Source: CAD feature listing. Evaluate the final solid. Frame: model axes, mm. Face numbers are marked on the shaded views. A direction names the side the tool comes from. Coordinates: 2 decimals unless noted, no trailing zeros. Write each loop counter-clockwise with the first axis right and the second up, starting at its lowest first coordinate (ties: lowest second). Pieces come first, ordered by that corner, then holes. Notation, with made-up numbers: (24.25, 86) -> (37.25, 86) arc R23 ccw to (37.25, 100) -> close; hole circle Ø3 at (12.5, 4). An arc over 180 degrees is marked (long way). One line per item, written item: value. Start each with the question number.
1. Mould query, pull axis Y, two halves, no side actions, for the marked faces 1, 2 and 3. Classes: released by +Y, released by -Y, zero draft, split by the parting line, or undercut.
2. Section query D-D, the plane z = 2.5. Output: boundary loops of the cut face in (x, y), and give its area (3 significant figures).
3. Section query C-C, the plane y = -0.9. Output: boundary loops of the cut face in (x, z), and give its area (3 significant figures).
4. Section query A-A, the plane z = 6.75. Output: boundary loops of the cut face in (x, y).
5. Line query: line 1 (Y direction, x = 0, z = 1.95); line 2 (Z direction, x = 1.1, y = -0.1); line 3 (X direction, y = 0.05, z = 3.75). Output: solid intervals per line, ascending.
6. Section query B-B, the plane x = -0.75. Output: boundary loops of the cut face in (y, z).
7. Access query for the marked faces 4, 5 and 6. Directions: +Z, -Z, +X, -X, +Y, -Y. A direction counts if a zero-diameter tool reaches every point of the face in a straight line with its end or side. Return the directions, or none.
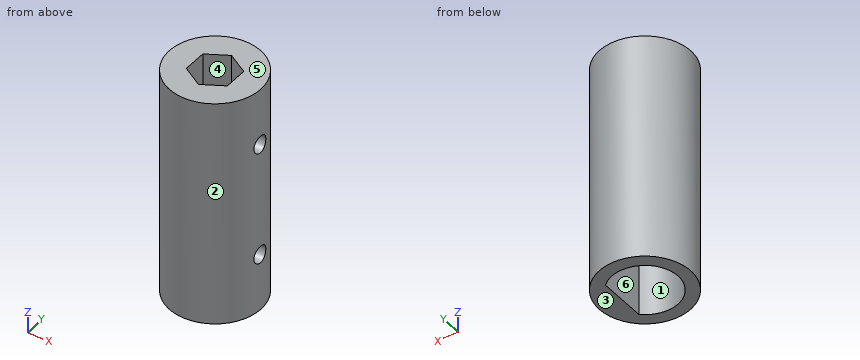
from build123d import *

# Parameters (mm, degrees)
MOTORSKE_R      = 2
MOTOR_DEPTH     = 5
AXISSKE_R       = 2
AXIS_DEPTH      = 5
SCREWHOLESKE_R  = 0.376260287
SCREWHOLE_DEPTH = 11.392304845


with BuildPart() as part:
    # MotorSke → Motor (new body)
    with BuildSketch(Plane.XY):
        Circle(MOTORSKE_R)
        with BuildLine():
            Line((1, 1.05), (1, -1.05))
            ThreePointArc((1, -1.05), (-1.45, 0), (1, 1.05))
        make_face(mode=Mode.SUBTRACT)
    extrude(amount=MOTOR_DEPTH)

    # AxisSke → Axis (add)
    with BuildSketch(Plane.XY.offset(5)):
        Circle(AXISSKE_R)
        Polygon((0, -1.039230485), (0.9, -0.519615242), (0.9, 0.519615242), (0, 1.039230485), (-0.9, 0.519615242), (-0.9, -0.519615242), align=None, mode=Mode.SUBTRACT)
    extrude(amount=AXIS_DEPTH)

    # ScrewHoleSke → ScrewHole (cut, through all)
    with BuildSketch(Plane(origin=(0, 0, 0), x_dir=(0, 0, -1), z_dir=(1, 0, 0))):
        with Locations(Location((-7.5, 0, 0), (0, 0, 180))):
            Circle(SCREWHOLESKE_R)
        with Locations(Location((-2.5, 0, 0), (0, 0, 180))):
            Circle(SCREWHOLESKE_R)
    extrude(amount=SCREWHOLE_DEPTH, mode=Mode.SUBTRACT)


solid = part.part
Computed values:
1. face 1: undercut
1. face 2: split by the parting line
1. face 3: zero draft
2. outline: (1, -1.05) arc R1.45 cw (long way) to (1, 1.05) -> (1, 0.38) -> (1.96, 0.38) arc R2 ccw (long way) to (1.96, -0.38) -> (1, -0.38) -> close
2. area: 5.87 mm²
3. outline: (-1.79, 0) -> (-1.14, 0) -> (-1.14, 5) -> (-0.24, 5) -> (-0.24, 10) -> (-1.79, 10) -> close; (0.24, 5) -> (1, 5) -> (1, 0) -> (1.79, 0) -> (1.79, 10) -> (0.24, 10) -> close
3. area: 22.6 mm²
4. outline: circle Ø4 at (0, 0); hole (-0.9, -0.52) -> (0, -1.04) -> (0.9, -0.52) -> (0.9, 0.52) -> (0, 1.04) -> (-0.9, 0.52) -> close
5. line 1: y = -2 to -1.45, 1.45 to 2
5. line 2: z = 0 to 2.14, 2.86 to 7.14, 7.86 to 10
5. line 3: x = -2 to -1.45, 1 to 2
6. outline: (-1.85, 0) -> (-1.24, 0) -> (-1.24, 5) -> (-0.61, 5) -> (-0.61, 10) -> (-1.85, 10) -> close; (0.61, 5) -> (1.24, 5) -> (1.24, 0) -> (1.85, 0) -> (1.85, 10) -> (0.61, 10) -> close
7. face 4: +Z, -Z
7. face 5: +Z, +X, -X, +Y, -Y
7. face 6: -Z
